Input: part model. Units: mm. Frame: model coordinates. A direction names the side the tool comes from. Round coordinates to 2 decimals unless told otherwise and drop trailing zeros. Loops run counter-clockwise (first coordinate to the right, second up) from the corner with the lowest first, then second, coordinate; pieces in that order, holes last. Notation, with made-up numbers: (-22, -40) - (16, -40) arc R12 ccw to (16, -31) - close; hole circle Ø4 at (68.25, 7). An arc over 180 degrees is marked (long way). Write each question's results on one line, items separated by ' | '.
from build123d import *

# Parameters (mm, degrees)
SALIENTE_EXTRUIR1_DEPTH = 3
CORTAR_EXTRUIR2_REACH   = 5


with BuildPart() as part:
    # Croquis1 → Saliente-Extruir1 (new body)
    with BuildSketch(Plane.XY):
        with BuildLine():
            Line((-6.614427743, -7.499956375), (0.826760185, -14.062554531))
            Line((0.826760185, -14.062554531), (-1.157568138, -16.312541443))
            Line((-1.157568138, -16.312541443), (-8.541931773, -9.80005827))
            ThreePointArc((-8.541931773, -9.80005827), (1.549305596, -24.879455682), (6.540102602, -7.434879356))
            Line((6.540102602, -7.434879356), (-0.901085326, -0.872281201))
            Line((-0.901085326, -0.872281201), (1.083242997, 1.377705712))
            Line((1.083242997, 1.377705712), (8.541627127, -5.20005827))
            ThreePointArc((8.541627127, -5.20005827), (-1.500302366, 9.886814088), (-6.614427743, -7.499956375))
        make_face()
    extrude(amount=SALIENTE_EXTRUIR1_DEPTH)

    # Croquis2 → Cortar-Extruir2 (cut, up to next)
    with BuildSketch(Plane(origin=(0, 0, 0), x_dir=(-1, 0, 0), z_dir=(0, 0, -1)), mode=Mode.PRIVATE) as cortar_extruir2_sk1:
        Polygon((-4.63280312, -13.586006872), (-0.132829295, -9.617350226), (-2.117157618, -7.367363313), (-6.617131443, -11.336019959), align=None)
    cortar_extruir2_tool1 = extrude(cortar_extruir2_sk1.sketch, amount=-CORTAR_EXTRUIR2_REACH, mode=Mode.PRIVATE) & part.part
    add(cortar_extruir2_tool1.solids().sort_by_distance((3.37498, -10.476685, 0))[0], mode=Mode.SUBTRACT)
    # Croquis2 → Cortar-Extruir2 (cut, up to next)
    with BuildSketch(Plane(origin=(0, 0, 0), x_dir=(-1, 0, 0), z_dir=(0, 0, -1)), mode=Mode.PRIVATE) as cortar_extruir2_sk2:
        Polygon((6.617131443, -3.664365257), (4.63280312, -1.414378344), (0.132829295, -5.38303499), (2.117157618, -7.633021903), align=None)
    cortar_extruir2_tool2 = extrude(cortar_extruir2_sk2.sketch, amount=-CORTAR_EXTRUIR2_REACH, mode=Mode.PRIVATE) & part.part
    add(cortar_extruir2_tool2.solids().sort_by_distance((-3.37498, -4.5237, 0))[0], mode=Mode.SUBTRACT)


solid = part.part
1. Section query A-A, the plane z = 2.45. Output: boundary loops of the cut face in (x, y), plus the area to 3 significant figures.
Answer:
outline: (-8.54, -9.8) arc R10 ccw (long way) to (6.54, -7.43) - (-0.9, -0.87) - (1.08, 1.38) - (8.54, -5.2) arc R10 ccw (long way) to (-6.61, -7.5) - (0.83, -14.06) - (-1.16, -16.31) - close; hole (-6.62, -3.66) - (-2.12, -7.63) - (-0.13, -5.38) - (-4.63, -1.41) - close; hole (0.13, -9.62) - (4.63, -13.59) - (6.62, -11.34) - (2.12, -7.37) - close | area: 487 mm^2
2. Section query C-C, the plane y = 0. Output: boundary loops of the cut face in (x, z).
Answer:
outline: (-10, 0) - (-0.13, 0) - (-0.13, 3) - (-10, 3) - close; (2.65, 0) - (10, 0) - (10, 3) - (2.65, 3) - close
3. Section query D-D, the plane x = -2.75. Output: boundary loops of the cut face in (y, z), plus the area to 3 significant figures.
Answer:
outline: (-24.61, 0) - (-14.91, 0) - (-14.91, 3) - (-24.61, 3) - close; (-10.91, 0) - (-7.07, 0) - (-7.07, 3) - (-10.91, 3) - close; (-3.07, 0) - (9.61, 0) - (9.61, 3) - (-3.07, 3) - close | area: 78.7 mm^2
4. Section query B-B, the plane x = -6. Output: boundary loops of the cut face in (y, z).
Answer:
outline: (-23, 0) - (-12.04, 0) - (-12.04, 3) - (-23, 3) - close; (-8.04, 0) - (-4.21, 0) - (-4.21, 3) - (-8.04, 3) - close; (-2.96, 0) - (8, 0) - (8, 3) - (-2.96, 3) - close
5. Contact query for flat-ended pins moving along their axis: pin 1 (1 mm diameter, centred on y = 1.5, z = 1, fed in from +X); pin 2 (1 mm diameter, centred on y = 1, z = 2, fed in from -X). Output: stop coordinate, or through.
Answer:
pin 1: x = 9.95 | pin 2: x = -9.99
6. Mould query, pull axis X, two halves, no side actions, for faces 3 (the flat face through (0, -7, 0)), 4 (the flat face through (-4.8, -13.1, 1.5)), 5 (the flat face through (2.87, -4.2, 1.48)), 6 (the cylindrical face through (1.234, -24.924, 1.479)). Classes: pulls with the +X half, pulls with the -X half, needs draft (parallel to the pull), parting line crosses it, or undercut.
Answer:
face 3: needs draft | face 4: undercut | face 5: undercut | face 6: parting line crosses it
7. Line query: line 1 (Y direction, x = -3.5, z = 1.6); line 2 (Y direction, x = 5, z = 1.4); line 3 (Y direction, x = 0.75, z = 2.6). Output: solid intervals per line, ascending. Write a range as [from, to].
Answer:
line 1: [-24.37, -14.25], [-10.25, -6.41], [-2.41, 9.37] | line 2: [-23.66, -13.17], [-9.91, -6.08], [-2.08, 8.66] | line 3: [-24.97, -14.15], [-13.99, -10.16], [-8.92, -2.33], [1, 9.97]
8. Set-up query: faces 1 (the flat face through (0, -7, 3)), 2 (the flat face through (1.11, -8.51, 1.48)). Return all of +Z, -Z, +X, -X, +Y, -Y with unobstructed straight access to the full face (end or side cutting, diameter ignored); none if empty.
Answer:
face 1: +Z, +X, -X, +Y, -Y | face 2: +Z, -Z
